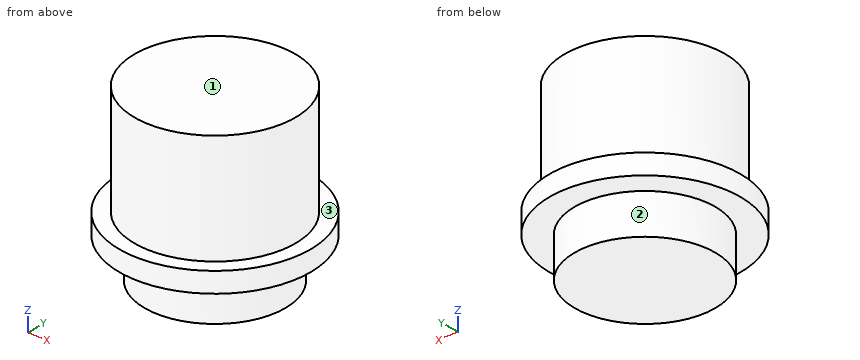
from build123d import *

# Parameters (mm, degrees)
SKETCH010_R             = 9.5
PAD008_DEPTH            = 2
SKETCH011_R             = 7
PAD009_DEPTH            = 4
SKETCH012_R             = 8
PAD010_DEPTH            = 11
BODY003_PLACEMENT_ANGLE = 180


with BuildPart() as part:
    # Sketch010 → Pad008 (new body)
    with BuildSketch(Plane.XY):
        Circle(SKETCH010_R)
    extrude(amount=PAD008_DEPTH)

    # Sketch011 (on Face3 of Pad008) → Pad009 (join)
    with BuildSketch(Plane.XY.offset(2)):
        Circle(SKETCH011_R)
    extrude(amount=PAD009_DEPTH)

    # Sketch012 (on Face2 of Pad009) → Pad010 (join)
    with BuildSketch(Plane(origin=(0, 0, 0), x_dir=(1, 0, 0), z_dir=(0, 0, -1))):
        Circle(SKETCH012_R)
    extrude(amount=PAD010_DEPTH)


with BuildPart() as part_1:
    # Body003 placement: moved
    add(part.part.moved(Location((25, 0, -2))).rotate(Axis((25, 0, -2), (0, 1, 0)), BODY003_PLACEMENT_ANGLE))


solid = part_1.part
Design review of the part built by this model. Coordinates are the model's own, in mm. Face numbers are marked on the shaded views. A direction names the side the tool comes from. Round coordinates to 2 decimals unless told otherwise and drop trailing zeros. Loops run counter-clockwise (first coordinate to the right, second up) from the corner with the lowest first, then second, coordinate; pieces in that order, holes last. Notation, with made-up numbers: (-20, 67) - (6, 67) arc R20 cw to (6, 88) - close; hole circle Ø2 at (-29, 20). An arc over 180 degrees is marked (long way). One line per question, with ' | ' between items.
1. For the marked faces 1, 2 and 3, list the 3-axis set-ups (+Z, -Z, +X, -X, +Y, -Y) from which the entire face can be reached by the end or side of a thin tool; tool diameter is ignored.
Results are:
face 1: +Z, +X, -X, +Y, -Y | face 2: -Z | face 3: +Z
2. We need section B-B, the plane y = 0. State the section outline as (x, z) points.
Results are:
outline: (15.5, -4) - (18, -4) - (18, -8) - (32, -8) - (32, -4) - (34.5, -4) - (34.5, -2) - (33, -2) - (33, 9) - (17, 9) - (17, -2) - (15.5, -2) - close
3. We need section D-D, the plane y = 7.5. State the section outline as (x, z) points.
Results are:
outline: (19.17, -4) - (30.83, -4) - (30.83, -2) - (27.78, -2) - (27.78, 9) - (22.22, 9) - (22.22, -2) - (19.17, -2) - close
4. For L1, parallel to Z at x = 24, y = 8.75; L2, parallel to Z at x = 24, y = -7; L3, parallel to X at y = 6.25, z = 3.75, list the stretches that pass through material, from the lowest coordinate up. Write a range as [from, to].
Results are:
L1: z = [-4, -2] | L2: z = [-4, 9] | L3: x = [20.01, 29.99]
5. We need section C-C, the plane z = -3. State the section outline as (x, y) points, and give its area (3 significant figures).
Results are:
outline: circle Ø19 at (25, 0) | area: 284 mm²
6. We need section A-A, the plane x = 25. State the section outline as (y, z) points, and give its area (3 significant figures).
Results are:
outline: (-9.5, -4) - (-7, -4) - (-7, -8) - (7, -8) - (7, -4) - (9.5, -4) - (9.5, -2) - (8, -2) - (8, 9) - (-8, 9) - (-8, -2) - (-9.5, -2) - close | area: 270 mm²
7. Clearance check with flat-ended pins moving along their axes: P1, Ø4, axis at y = -6.5, z = -5, coming from the +X side; P2, Ø3, axis at y = -1, z = 4, coming from the -X side; P3, Ø5, axis at x = 17.5, z = -2, coming from the +Y side. State where each tip first meets the part, or that it passes through.
Results are:
P1: stops at x = 33.22 | P2: stops at x = 17 | P3: stops at y = 8.08
